Read the model definition and answer for the solid it produces. Units are mm, in the model's axes. A direction names the side the tool comes from. Give positions to 0.01 mm unless a question says otherwise; leave off trailing zeros. Write each loop counter-clockwise with the first axis right and the second up, starting at its lowest first coordinate (ties: lowest second). Pieces come first, ordered by that corner, then holes. Notation, with made-up numbers: M 24,68 L 39,68 A27 cw 39,106 Z; hole C -14,4.25 d1. An arc over 180 degrees is marked long. Put each result on its own line as item: value.
from build123d import *

# Parameters (mm, degrees)
BOSS_EXTRUDE3_DEPTH = 2
BOSS_EXTRUDE4_DEPTH = 10
BOSS_EXTRUDE5_DEPTH = 5
SKETCH11_W          = 2.5
SKETCH11_H          = 5.612132728
BOSS_EXTRUDE7_DEPTH = 1.65
FILLET2_R           = 1
SKETCH12_W          = 7.5
SKETCH12_H          = 16.75
CUT_EXTRUDE1_DEPTH  = 2
SKETCH17_W          = 1.5
SKETCH17_H          = 14.5
BOSS_EXTRUDE8_DEPTH = 3
SKETCH18_R          = 2.5
SKETCH18_R_2        = 1.5
BOSS_EXTRUDE9_DEPTH = 8
FILLET3_R           = 2
FILLET4_R           = 1


with BuildPart() as part:
    # Sketch4 → Boss-Extrude3 (new body)
    with BuildSketch(Plane(origin=(0, 0, 0), x_dir=(1, 0, 0), z_dir=(0, 1, 0))):
        with BuildLine():
            ThreePointArc((37.3, 17.020869543), (-41, 0), (37.3, -17.020869543))
            ThreePointArc((37.3, -17.020869543), (46, 0), (37.3, 17.020869543))
        make_face()
    extrude(amount=BOSS_EXTRUDE3_DEPTH)

    # Sketch4<5> → Boss-Extrude4 (add)
    with BuildSketch(Plane(origin=(0, 0, 0), x_dir=(1, 0, 0), z_dir=(0, 1, 0))):
        with BuildLine():
            ThreePointArc((36.5, 16.363068172), (-40, 0), (36.5, -16.363068172))
            ThreePointArc((36.5, -16.363068172), (45, 0), (36.5, 16.363068172))
        make_face()
        with BuildLine():
            ThreePointArc((35.3, -15.36749817), (43.5, 0), (35.3, 15.36749817))
            ThreePointArc((35.3, 15.36749817), (-38.5, 0), (35.3, -15.36749817))
        make_face(mode=Mode.SUBTRACT)
    extrude(amount=BOSS_EXTRUDE4_DEPTH)

    # Sketch4<6> → Boss-Extrude5 (add)
    with BuildSketch(Plane(origin=(0, 0, 0), x_dir=(1, 0, 0), z_dir=(0, 1, 0))):
        with BuildLine():
            ThreePointArc((37.3, 17.020869543), (-41, 0), (37.3, -17.020869543))
            ThreePointArc((37.3, -17.020869543), (46, 0), (37.3, 17.020869543))
        make_face()
        with BuildLine():
            ThreePointArc((36.5, -16.363068172), (45, 0), (36.5, 16.363068172))
            ThreePointArc((36.5, 16.363068172), (-40, 0), (36.5, -16.363068172))
        make_face(mode=Mode.SUBTRACT)
    extrude(amount=BOSS_EXTRUDE5_DEPTH)

    # Sketch11 → Boss-Extrude7 (add)
    with BuildSketch(Plane(origin=(0, 10, 0), x_dir=(1, 0, 0), z_dir=(0, 1, 0))):
        with Locations((45, 0)):
            Rectangle(SKETCH11_W, SKETCH11_H)
    extrude(amount=-BOSS_EXTRUDE7_DEPTH)

    # Fillet2
    fillet2_edges = [part.edges().sort_by_distance(p)[0] for p in [
        (46.25, 8.35, 0),
    ]]
    fillet(fillet2_edges, radius=FILLET2_R)

    # Sketch12 → Cut-Extrude1 (cut)
    with BuildSketch(Plane.XZ):
        with Locations((-12.25, 0)):
            Rectangle(SKETCH12_W, SKETCH12_H)
    extrude(amount=-CUT_EXTRUDE1_DEPTH, mode=Mode.SUBTRACT)

    # Sketch17 → Boss-Extrude8 (add)
    with BuildSketch(Plane(origin=(0, 2, 0), x_dir=(1, 0, 0), z_dir=(0, 1, 0))):
        Polygon((-5.625, 0), (-5.625, -7.25), (-4.125, -7.25), (-4.125, 7.25), (-5.625, 7.25), align=None)
        with Locations((-19.625, 0)):
            Rectangle(SKETCH17_W, SKETCH17_H)
    extrude(amount=BOSS_EXTRUDE8_DEPTH)

    # Sketch18 → Boss-Extrude9 (add)
    # profile 1 of 2: a face of its own
    with BuildSketch(Plane(origin=(0, 2, 0), x_dir=(1, 0, 0), z_dir=(0, 1, 0))):
        with Locations(Location((-12.25, -18.5, 0), (0, 0, 270))):
            Circle(SKETCH18_R)
        with Locations(Location((-12.25, -18.5, 0), (0, 0, 270))):
            Circle(SKETCH18_R_2, mode=Mode.SUBTRACT)
    # profile 2 of 2: a face of its own
    with BuildSketch(Plane(origin=(0, 2, 0), x_dir=(1, 0, 0), z_dir=(0, 1, 0))):
        with Locations(Location((-12.25, 18.5, 0), (0, 0, 270))):
            Circle(SKETCH18_R)
        with Locations(Location((-12.25, 18.5, 0), (0, 0, 270))):
            Circle(SKETCH18_R_2, mode=Mode.SUBTRACT)
    extrude(amount=BOSS_EXTRUDE9_DEPTH)

    # Fillet3
    fillet3_edges = [part.edges().sort_by_distance(p)[0] for p in [
        (46, 0, 0),
        (-41, 0, 0),
    ]]
    fillet(fillet3_edges, radius=FILLET3_R)

    # Fillet4
    fillet4_edges = [part.edges().sort_by_distance(p)[0] for p in [
        (43.5, 2, 0),
        (-38.5, 2, 0),
    ]]
    fillet(fillet4_edges, radius=FILLET4_R)


solid = part.part
(1) Section A-A on y = 7 is taken. Determine the outline of the cut face in (x, z).
Result:
outline: C -12.25,-18.5 d5; C -12.25,18.5 d5; M 36.5,-16.36 A20 ccw 36.5,16.36 A40 ccw long Z; hole C -12.25,-18.5 d3; hole C -12.25,18.5 d3; hole M 35.3,-15.37 A18.5 ccw 35.3,15.37 A38.5 ccw long Z
(2) For a pull along X with two mould halves and no side action, classify faces 1 (the face through (-13, 10, 20)), 2 (the face through (-39.97, 7.46, -1.52)), 3 (the face through (-20.375, 3, 0)), 4 (the face through (-18.875, 3, 0)) as +X half, -X half, draft (parallel to the pull), parting line (faces both ways), or undercut.
Result:
face 1: draft
face 2: parting line
face 3: undercut
face 4: undercut
(3) Straight lines are drawn through the part: line 1 along X through (y, z) = (8, 18.5); line 2 along Y through (x, z) = (9, 27.5); line 3 along Z through (x, y) = (10.5, 5.5). For each, find the intervals that lie inside material, in ascending order. Write a range as from..to.
Result:
line 1: x = -35.46..-33.76, -14.75..-13.75, -10.75..-9.75, 33.76..35.46
line 2: y = 0..2
line 3: z = -38.6..-37.04, 37.04..38.6
(4) Which of the six approach directions +Z, -Z, +X, -X, +Y, -Y give full straight-line access (tool end or side, diameter ignored) to faces 5 (the face through (2, 0, -1)), 6 (the face through (-12, 2, -19)), 7 (the face through (-16, 1, 0))?
Result:
face 5: +Z, -Z, +X, -X, -Y
face 6: +Y
face 7: +Y, -Y
(5) Given pin 1 Ø3 at (y, z) = (2, 4.5) entering from -X; pin 2 Ø1.2 at (x, y) = (-5, 3) entering from -Z; pin 3 Ø1.5 at (y, z) = (2, 20.5) entering from +X, each flat-ended and moving along its own axis, determine where each tip first touches the part or whether it passes through.
Result:
pin 1: stops at x = -40.89
pin 2: stops at z = -40.76
pin 3: stops at x = 35.93
